For this review, take the finished solid that the model builds, in its own axes (mm). Face numbers are marked on the shaded views. A direction names the side the tool comes from. Coordinates: 2 decimals unless noted, no trailing zeros. Order: outer loops, then holes, each group sorted by start corner. A loop starts at its lowest first (then second) coordinate and runs counter-clockwise, first axis right, second up. Notation, with made-up numbers: (-38.75, -3) - (-16.75, -3) arc R26 cw to (-16.75, 20) - close; hole circle Ø11 at (32, 10.25). An arc over 180 degrees is marked (long way). One line per item, written item: value. Start each with the question number.
(1) Consider section C-C on x = 1.75. Write out the cut boundary in (y, z), then the cut area to 3 significant figures.
(2) To check wall thickness, follow line 1 along X through (y, z) = (-0.9, 1.65); line 2 along Z through (x, y) = (3, -0.45); line 3 along Y through (x, z) = (8.5, 1.1). State the ranges of each line that lie inside material, in increasing order.
(3) For the marked faces 1, 2 and 3, list the 3-axis set-ups (+Z, -Z, +X, -X, +Y, -Y) from which the entire face can be reached by the end or side of a thin tool; tool diameter is ignored.
(4) Consider section B-B on y = 0. Write out the cut boundary in (x, z), then the cut area to 3 significant figures.
(5) Consider section D-D on x = 6. Write out the cut boundary in (y, z), then the cut area to 3 significant figures.
(6) Clearance check with flat-ended pins moving along their axes: pin 1 (0.7 mm diameter, centred on x = 7, z = 0.5, fed in from -Y); pin 2 (1.5 mm diameter, centred on x = 9, y = 0.5, fed in from +Z); pin 3 (3 mm diameter, centred on x = 8.5, y = -1.5, fed in from -Z). State where each tip first meets the part, or that it passes through.
(7) Consider section A-A on z = 0. Write out the cut boundary in (x, y).
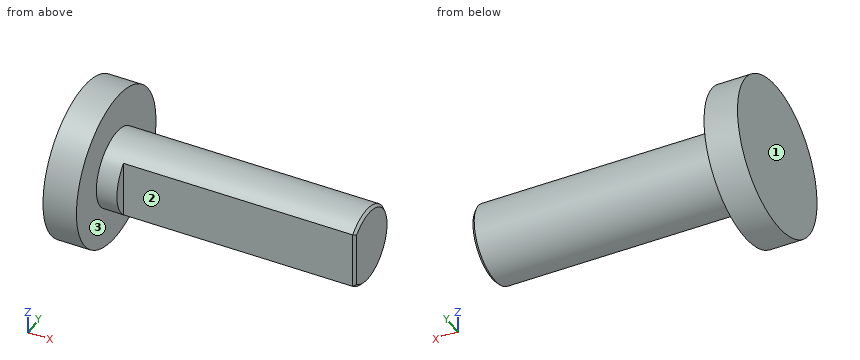
```python
from build123d import *

# Parameters (mm, degrees)
SKIZZE2_W                       = 2.236067978
SKIZZE2_H                       = 0.5
SCHNITT_LINEAR_AUSTRAGEN1_DEPTH = 9
FASE1_SIZE                      = 0.1


with BuildPart() as part:
    # Skizze1 → Rotation1 (revolve)
    with BuildSketch(Plane.XY, mode=Mode.PRIVATE) as rotation1_sk:
        Polygon((0, 0), (0, 3), (1.3, 3), (1.3, 1.5), (11.1, 1.5), (11.1, 0), align=None)
    revolve(rotation1_sk.sketch.rotate(Axis((0, 0, 0), (1, 0, 0)), 90), axis=Axis((0, 0, 0), (1, 0, 0)))

    # Skizze2 → Schnitt-Linear austragen1 (cut)
    with BuildSketch(Plane(origin=(11.1, 0, 0), x_dir=(0, 0, -1), z_dir=(1, 0, 0))):
        with Locations((0, -1.25)):
            Rectangle(SKIZZE2_W, SKIZZE2_H)
    extrude(amount=-SCHNITT_LINEAR_AUSTRAGEN1_DEPTH, mode=Mode.SUBTRACT)

    # Fase1
    fase1_edges = [part.edges().sort_by_distance(p)[0] for p in [
        (11.1, 1.401258538, -0.535233135),
        (11.1, -1, 0),
    ]]
    chamfer(fase1_edges, length=FASE1_SIZE)


solid = part.part
```
Geometry check:
1. outline: circle Ø3 at (0, 0)
1. area: 7.07 mm^2
2. line 1: x = 0 to 1.3
2. line 2: z = -1.43 to 1.43
2. line 3: y = -1 to 1.02
3. face 1: +Z, -Z, -X, +Y, -Y
3. face 2: +Z, -Z, +X, -Y
3. face 3: +X
4. outline: (0, -3) - (1.3, -3) - (1.3, -1.5) - (11, -1.5) - (11.1, -1.4) - (11.1, 1.4) - (11, 1.5) - (1.3, 1.5) - (1.3, 3) - (0, 3) - close
4. area: 37.2 mm^2
5. outline: (-1, -1.12) arc R1.5 ccw (long way) to (-1, 1.12) - close
5. area: 6.29 mm^2
6. pin 1: stops at y = -1
6. pin 2: stops at z = 1.5
6. pin 3: stops at z = -1.5
7. outline: (0, -3) - (1.3, -3) - (1.3, -1.5) - (2.1, -1.5) - (2.1, -1) - (11, -1) - (11.1, -0.9) - (11.1, 1.4) - (11, 1.5) - (1.3, 1.5) - (1.3, 3) - (0, 3) - close
